The listing builds one solid part. Answer for the finished solid, in the listing's coordinates (mm). Face numbers are marked on the shaded views. A direction names the side the tool comes from. Give positions to 0.01 mm unless a question says otherwise; leave off trailing zeros. Order: outer loops, then holes, each group sorted by start corner. A loop starts at its lowest first (then second) coordinate and runs counter-clockwise, first axis right, second up. Notation, with made-up numbers: (-29.75, -18.75) - (13.25, -18.75) arc R9 ccw to (13.25, -4.75) - close; hole circle Ø2 at (38.25, -18). An arc over 180 degrees is marked (long way). Answer as a JSON object with one key per item and string values. Group by question number.
Q1. A cutting plane is placed at A-A, the plane x = 0. Give the vertices of the cut face in (y, z), and give its area (3 significant figures).
Q2. The mould has two halves that part along X. Classify the marked faces 1 and 2: released by +X, released by -X, zero draft, split by the parting line, or undercut.
Q3. Consider line 1 (Y direction, x = 40, z = -1.75); line 2 (Y direction, x = 97.5, z = 6.25); line 3 (Y direction, x = 0, z = 2.1). Determine where each line is inside the solid, lowest interval first.
Q4. A cutting plane is placed at C-C, the plane z = 9.5. Give the vertices of the cut face in (x, y), and give its area (3 significant figures).
Q5. A cutting plane is placed at B-B, the plane y = 0. Give the vertices of the cut face in (x, z).
Q6. For the marked faces 3 and 4, determine the directions among +Z, -Z, +X, -X, +Y, -Y from which every point of the face is accessible in a straight line to the end or side of a thin tool.
Q7. Given pin 1 (17 mm diameter, centred on x = 28.5, y = 112.5, fed in from -Z); pin 2 (2 mm diameter, centred on x = -94, y = 12.5, fed in from +Z), each flat-ended and moving along its own axis, determine where each tip first touches the part or whether it passes through.
Q8. A cutting plane is placed at D-D, the plane y = -66. Give the vertices of the cut face in (x, z).
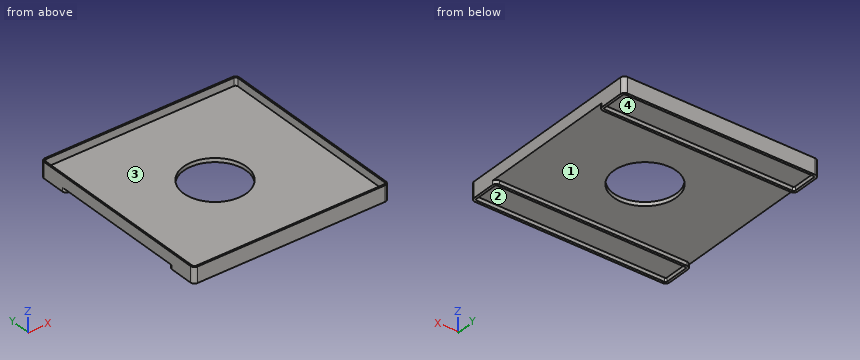
from build123d import *

# Parameters (mm, degrees)
F1_DEPTH = 5
F3_DEPTH = 10
F4_R     = 40
F5_DEPTH = 5.001
F7_DEPTH = 5


# Not quite as in the source:
# - a pattern or mirror of a feature is missing from the dataset's text; its kind, count and spacing are read off the source's solid


with BuildPart() as f1:
    # F0 (on Top) → F1 (new body)
    with BuildSketch(Plane.XY):
        with BuildLine():
            ThreePointArc((125, 120), (123.5355339059, 123.5355339059), (120, 125))
            Line((120, 125), (-120, 125))
            ThreePointArc((-120, 125), (-123.5355339059, 123.5355339059), (-125, 120))
            Line((-125, 120), (-125, -120))
            ThreePointArc((-125, -120), (-123.5355339059, -123.5355339059), (-120, -125))
            Line((-120, -125), (120, -125))
            ThreePointArc((120, -125), (123.5355339059, -123.5355339059), (125, -120))
            Line((125, -120), (125, 120))
        make_face()
    extrude(amount=F1_DEPTH)

    # F2 (on face) → F3 (join)
    with BuildSketch(Plane.XY.offset(5)):
        with BuildLine():
            ThreePointArc((-120, 125), (-123.5355339059, 123.5355339059), (-125, 120))
            Line((-125, 120), (-125, -120))
            ThreePointArc((-125, -120), (-123.5355339059, -123.5355339059), (-120, -125))
            Line((-120, -125), (120, -125))
            ThreePointArc((120, -125), (123.5355339059, -123.5355339059), (125, -120))
            Line((125, -120), (125, 120))
            ThreePointArc((125, 120), (123.5355339059, 123.5355339059), (120, 125))
            Line((120, 125), (-120, 125))
        make_face()
        with BuildLine():
            Line((-120, 123), (120, 123))
            ThreePointArc((120, 123), (122.1213203436, 122.1213203436), (123, 120))
            Line((123, 120), (123, -120))
            ThreePointArc((123, -120), (122.1213203436, -122.1213203436), (120, -123))
            Line((120, -123), (-120, -123))
            ThreePointArc((-120, -123), (-122.1213203436, -122.1213203436), (-123, -120))
            Line((-123, -120), (-123, 120))
            ThreePointArc((-123, 120), (-122.1213203436, 122.1213203436), (-120, 123))
        make_face(mode=Mode.SUBTRACT)
    extrude(amount=F3_DEPTH)

    # F4 (on face) → F5 (cut, through all)
    with BuildSketch(Plane.XY.offset(5)):
        Circle(F4_R)
    extrude(amount=-F5_DEPTH, mode=Mode.SUBTRACT)

    # F6 (on face) → F7 (join)
    with BuildSketch(Plane(origin=(0, 0, 0), x_dir=(1, 0, 0), z_dir=(0, 0, -1))):
        with BuildLine():
            ThreePointArc((-120, 125), (-123.5355339059, 123.5355339059), (-125, 120))
            Line((-125, 120), (-125, 90))
            ThreePointArc((-125, 90), (-123.5355339059, 86.4644660941), (-120, 85))
            Line((-120, 85), (120, 85))
            ThreePointArc((120, 85), (123.5355339059, 86.4644660941), (125, 90))
            Line((125, 90), (125, 120))
            ThreePointArc((125, 120), (123.5355339059, 123.5355339059), (120, 125))
            Line((120, 125), (-120, 125))
        make_face()
        with BuildLine():
            Line((-122, 90), (-122, 120))
            ThreePointArc((-122, 120), (-121.4142135624, 121.4142135624), (-120, 122))
            Line((-120, 122), (120, 122))
            ThreePointArc((120, 122), (121.4142135624, 121.4142135624), (122, 120))
            Line((122, 120), (122, 90))
            ThreePointArc((122, 90), (121.4142135624, 88.5857864376), (120, 88))
            Line((120, 88), (-120, 88))
            ThreePointArc((-120, 88), (-121.4142135624, 88.5857864376), (-122, 90))
        make_face(mode=Mode.SUBTRACT)
    f7 = extrude(amount=F7_DEPTH)

    # F7_copies: F7 across plane
    add(f7.mirror(Plane.ZX))


solid = f1.part
Reply:
{
 "1": {"outline": "(-125, -5) - (-122, -5) - (-122, 0) - (-88, 0) - (-88, -5) - (-85, -5) - (-85, 0) - (-40, 0) - (-40, 5) - (-123, 5) - (-123, 15) - (-125, 15) - close; (40, 0) - (85, 0) - (85, -5) - (88, -5) - (88, 0) - (122, 0) - (122, -5) - (125, -5) - (125, 15) - (123, 15) - (123, 5) - (40, 5) - close", "area": "950 mm^2"},
 "2": {"face 1": "zero draft", "face 2": "undercut"},
 "3": {"line 1": "y = -125 to -122, -88 to -85, 85 to 88, 122 to 125", "line 2": "y = -125 to -123, 123 to 125", "line 3": "y = -125 to -40, 40 to 125"},
 "4": {"outline": "(-125, -120) arc R5 ccw to (-120, -125) - (120, -125) arc R5 ccw to (125, -120) - (125, 120) arc R5 ccw to (120, 125) - (-120, 125) arc R5 ccw to (-125, 120) - close; hole (-123, -120) arc R3 ccw to (-120, -123) - (120, -123) arc R3 ccw to (123, -120) - (123, 120) arc R3 ccw to (120, 123) - (-120, 123) arc R3 ccw to (-123, 120) - close", "area": "1,970 mm^2"},
 "5": {"outline": "(-125, 0) - (-40, 0) - (-40, 5) - (-123, 5) - (-123, 15) - (-125, 15) - close; (40, 0) - (125, 0) - (125, 15) - (123, 15) - (123, 5) - (40, 5) - close"},
 "6": {"face 3": "+Z", "face 4": "-Z"},
 "7": {"pin 1": "stops at z = 0", "pin 2": "stops at z = 5"},
 "8": {"outline": "(-125, 0) - (125, 0) - (125, 15) - (123, 15) - (123, 5) - (-123, 5) - (-123, 15) - (-125, 15) - close"}
}
